Design review of the part built by this model. Coordinates are the model's own, in mm. A direction names the side the tool comes from. Round coordinates to 2 decimals unless told otherwise and drop trailing zeros. Write each loop counter-clockwise with the first axis right and the second up, starting at its lowest first coordinate (ties: lowest second). Pieces come first, ordered by that corner, then holes. Notation, with made-up numbers: (32.25, 68.25) -> (38.25, 68.25) arc R29 cw to (38.25, 92.25) -> close; hole circle Ø4 at (24, 47.5). An arc over 180 degrees is marked (long way). Write item = value, one per line. Start each with the question number.
Item 1: For pin 1 Ø6 at (x, z) = (-40, 5.5) entering from -Y, flat-tipped, find the tip position at first contact; note if it passes through.
Item 2: Add section A-A, the plane x = -85.5. State the section outline as (y, z) points.
Item 3: Mouldability with a two-part tool opening along Z and no side actions: class faces 1 (the flat face through (-90, -1.426, 6)), 2 (the flat face through (-15, 10, 3)), 3 (the flat face through (15.724, 0.354, 8.825)), 4 (the flat face through (16.5, 2, 5)) as released by +Z, released by -Z, zero draft, split by the parting line, or undercut.
Item 4: Add section B-B, the plane x = -58.5. State the section outline as (y, z) points, then the cut area to 3 significant figures.
Item 5: To check wall thickness, follow L1, parallel to Y at x = -85, z = 7; L2, parallel to X at y = 12.75, z = 5.5; L3, parallel to X at y = 5.75, z = 5.25. State the ranges of each line that lie inside material, in increasing order.
Item 6: Machinability: for faces 5 (the flat face through (-90.28, -6.825, 4.445)), 6 (the flat face through (15.68, 6.56, 5.17)), 7 (the cylindrical face through (-47.021, 5.456, 6.912)), which of the approach directions +Z, -Z, +X, -X, +Y, -Y give a long, thin tool a straight path to every point of the face, cutting with its end or side? Answer none if there is none.
from build123d import *

# Parameters (mm, degrees)
ESQUISSE1_W                   = 65
ESQUISSE1_H                   = 20.233469585
BOSS_EXTRU_9_DEPTH            = 12
BOSS_EXTRU_10_DEPTH           = 7
BOSS_EXTRU_11_DEPTH           = 12
ESQUISSE1_18_W                = 25
ESQUISSE1_18_H                = 20.233469585
BOSS_EXTRU_12_DEPTH           = 2
ENL_V_MAT_EXTRU_5_DEPTH       = 102.658790864
ENL_V_MAT_EXTRU_5_DEPTH_BACK  = 102.658790864
ESQUISSE3_R                   = 4
ESQUISSE3_R_2                 = 2
ENL_V_MAT_EXTRU_6_DEPTH       = 2
ENL_V_MAT_EXTRU_13_DEPTH      = 9
ENL_V_MAT_EXTRU_15_DEPTH      = 38
ENL_V_MAT_EXTRU_15_DEPTH_BACK = 53
ESQUISSE12_R                  = 2
ENL_V_MAT_EXTRU_16_DEPTH      = 16.5
ENL_V_MAT_EXTRU_16_DEPTH_BACK = 46.5


with BuildPart() as part:
    # Esquisse1 → Boss.-Extru.9 (new body)
    with BuildSketch(Plane.XY):
        with Locations((-15.027863484, 3.457446809)):
            Rectangle(ESQUISSE1_W, ESQUISSE1_H)
        with BuildLine():
            ThreePointArc((7.569520453, -4.659287984), (15.686255246, 3.457446809), (7.569520453, 11.574181601))
            Line((7.569520453, 11.574181601), (-37.62524742, 11.574181601))
            ThreePointArc((-37.62524742, 11.574181601), (-45.741982213, 3.457446809), (-37.62524742, -4.659287984))
            Line((-37.62524742, -4.659287984), (7.569520453, -4.659287984))
        make_face(mode=Mode.SUBTRACT)
    extrude(amount=BOSS_EXTRU_9_DEPTH)

    # Esquisse1_14 → Boss.-Extru.10 (add)
    with BuildSketch(Plane.XY):
        with BuildLine():
            Line((-37.62524742, -4.659287984), (7.569520453, -4.659287984))
            ThreePointArc((7.569520453, -4.659287984), (15.686255246, 3.457446809), (7.569520453, 11.574181601))
            Line((7.569520453, 11.574181601), (-37.62524742, 11.574181601))
            ThreePointArc((-37.62524742, 11.574181601), (-45.741982213, 3.457446809), (-37.62524742, -4.659287984))
        make_face()
        with BuildLine():
            ThreePointArc((7.569520453, -2.542553191), (13.569520453, 3.457446809), (7.569520453, 9.457446809))
            Line((7.569520453, 9.457446809), (-37.62524742, 9.457446809))
            ThreePointArc((-37.62524742, 9.457446809), (-43.62524742, 3.457446809), (-37.62524742, -2.542553191))
            Line((-37.62524742, -2.542553191), (7.569520453, -2.542553191))
        make_face(mode=Mode.SUBTRACT)
    extrude(amount=BOSS_EXTRU_10_DEPTH)



with BuildPart() as body_2:
    # Esquisse1_17 → Boss.-Extru.11 (new body)
    with BuildSketch(Plane.XY):
        Polygon((-72.527863484, 13.574181601), (-86.527863484, 13.574181601), (-86.527863484, 5.187945625), (-100.031251885, 5.187945625), (-100.031251885, -0.175818399), (-75.527863484, -0.175818399), (-75.527863484, -1.425818399), (-100.031251885, -1.425818399), (-100.031251885, -7.810998677), (-86.527863484, -7.810998677), (-86.527863484, -6.659287984), (-72.527863484, -6.659287984), align=None)
    extrude(amount=BOSS_EXTRU_11_DEPTH)


with BuildPart() as part_1:
    add(part.part)

    add(body_2.part)  # Boss.-Extru.12 merges body 2
    # Esquisse1_18 → Boss.-Extru.12 (add)
    with BuildSketch(Plane.XY):
        with Locations((-60.027863484, 3.457446809)):
            Rectangle(ESQUISSE1_18_W, ESQUISSE1_18_H)
    extrude(amount=BOSS_EXTRU_12_DEPTH)

    # Esquisse3 → Enl_v. mat.-Extru.5 (cut, two sides: drawn at the far end of the back side and taken through both)
    with BuildSketch(Plane(origin=(0, 0, 0), x_dir=(1, 0, 0), z_dir=(0, 1, 0)).offset(-ENL_V_MAT_EXTRU_5_DEPTH_BACK)):
        with Locations(Location((-79.75826264, -6.22368636, 0), (0, 0, 270))):
            Circle(ESQUISSE3_R)
        with Locations(Location((-93.295048271, -6.22368636, 0), (0, 0, 270))):
            Circle(ESQUISSE3_R_2)
    extrude(amount=ENL_V_MAT_EXTRU_5_DEPTH + ENL_V_MAT_EXTRU_5_DEPTH_BACK, mode=Mode.SUBTRACT)

    # Esquisse4 → Enl_v. mat.-Extru.6 (cut)
    with BuildSketch(Plane.XZ.offset(7.810998677)):
        Polygon((-91.278888912, 2.721053811), (-89.253599824, 6.218415309), (-91.269759184, 9.721047858), (-95.311207631, 9.726318909), (-97.336496718, 6.228957411), (-95.320337359, 2.726324862), align=None)
    extrude(amount=-ENL_V_MAT_EXTRU_6_DEPTH, mode=Mode.SUBTRACT)

    # Esquisse9 → Enl_v. mat.-Extru.13 (cut)
    with BuildSketch(Plane.XY.offset(12)):
        with BuildLine():
            Line((-37.527863484, 11.557446809), (7.472136516, 11.557446809))
            ThreePointArc((7.472136516, 11.557446809), (15.572136516, 3.457446809), (7.472136516, -4.642553191))
            Line((7.472136516, -4.642553191), (-37.527863484, -4.642553191))
            ThreePointArc((-37.527863484, -4.642553191), (-45.627863484, 3.457446809), (-37.527863484, 11.557446809))
        make_face()
    extrude(amount=-ENL_V_MAT_EXTRU_13_DEPTH, mode=Mode.SUBTRACT)

    # Esquisse12 → Enl_v. mat.-Extru.15 (cut, two sides: drawn at the far end of the back side and taken through both)
    with BuildSketch(Plane(origin=(0, 0, 0), x_dir=(0, 0, -1), z_dir=(1, 0, 0)).offset(-ENL_V_MAT_EXTRU_15_DEPTH_BACK)):
        with Locations(Location((-7, 3.457446809, 0), (0, 0, 270))):
            Circle(ESQUISSE12_R)
    extrude(amount=ENL_V_MAT_EXTRU_15_DEPTH + ENL_V_MAT_EXTRU_15_DEPTH_BACK, mode=Mode.SUBTRACT)

    # Esquisse13 → Enl_v. mat.-Extru.16 (cut, two sides: drawn at the far end of the back side and taken through both)
    with BuildSketch(Plane(origin=(0, 0, 0), x_dir=(0, 0, -1), z_dir=(1, 0, 0)).offset(-ENL_V_MAT_EXTRU_16_DEPTH_BACK)):
        Polygon((-7, -0.69947513), (-3.4, 1.378985839), (-3.4, 5.535907778), (-7, 7.614368747), (-10.6, 5.535907778), (-10.6, 1.378985839), align=None)
    extrude(amount=ENL_V_MAT_EXTRU_16_DEPTH + ENL_V_MAT_EXTRU_16_DEPTH_BACK, mode=Mode.SUBTRACT)


solid = part_1.part
Result set:
q1.pin_1 = -6.66
q2.outline = (-6.66, 0) -> (-1.43, 0) -> (-1.43, 12) -> (-6.66, 12) -> close; (-0.18, 0) -> (13.57, 0) -> (13.57, 12) -> (-0.18, 12) -> close
q3.face_1 = zero draft
q3.face_2 = released by +Z
q3.face_3 = undercut
q3.face_4 = undercut
q4.outline = (-6.66, 0) -> (13.57, 0) -> (13.57, 2) -> (-6.66, 2) -> close
q4.area = 40.5 mm²
q5.L1 = -6.66 to -1.43, -0.18 to 13.57
q5.L2 = -86.53 to -83.69, -75.82 to -72.53, -47.53 to 17.47
q5.L3 = -86.53 to -83.64, -75.88 to -72.53, -47.53 to -46.5, 16.5 to 17.47
q6.face_5 = -Y
q6.face_6 = none
q6.face_7 = +X
